Source: CAD feature listing. Evaluate the final solid. Frame: model axes, mm. A direction names the side the tool comes from. Give positions to 0.01 mm unless a question says otherwise; leave off trailing zeros. Order: outer loops, then holes, each group sorted by start corner. A loop starts at its lowest first (then second) coordinate and runs counter-clockwise, first axis right, second up. Notation, with made-up numbers: M -12,81.25 L 33,81.25 A18 cw 33,107.25 Z; hole C 45,89.5 d11. An arc over 180 degrees is marked long. Return JSON: item names as keys, results as strings.
from build123d import *

# Parameters (mm, degrees)
SKETCH1_R           = 4
BOSS_EXTRUDE1_DEPTH = 10
SKETCH2_W           = 2
SKETCH2_H           = 10
CUT_EXTRUDE1_DEPTH  = 10
SKETCH3_R           = 1.5
CUT_EXTRUDE2_DEPTH  = 10
SKETCH4_W           = 4
SKETCH4_H           = 9
CUT_EXTRUDE3_DEPTH  = 10
SKETCH5_W           = 30
SKETCH5_H           = 10
BOSS_EXTRUDE2_DEPTH = 5
SKETCH6_R           = 8
CUT_EXTRUDE4_DEPTH  = 48
SKETCH7_R           = 6
CUT_EXTRUDE5_DEPTH  = 65
SKETCH8_R           = 6
CUT_EXTRUDE6_DEPTH  = 16
BOSS_EXTRUDE3_DEPTH = 15
SKETCH10_R          = 6
CUT_EXTRUDE7_DEPTH  = 6
FILLET1_R           = 5
FILLET2_R           = 5


with BuildPart() as part:
    # Sketch1 → Boss-Extrude1 (new body)
    with BuildSketch(Plane.XY):
        Polygon((0, 0), (30, 0), (30, -84), (-35, -84), (-35, -52), (0, -52), align=None)
        with Locations((20, -39)):
            Circle(SKETCH1_R, mode=Mode.SUBTRACT)
        with Locations((20, -67)):
            Circle(SKETCH1_R, mode=Mode.SUBTRACT)
    extrude(amount=BOSS_EXTRUDE1_DEPTH)

    # Sketch2 → Cut-Extrude1 (cut)
    with BuildSketch(Plane.XY.offset(10)):
        with Locations((29, -15)):
            Rectangle(SKETCH2_W, SKETCH2_H)
    extrude(amount=-CUT_EXTRUDE1_DEPTH, mode=Mode.SUBTRACT)

    # Sketch3 → Cut-Extrude2 (cut)
    with BuildSketch(Plane(origin=(30, 0, 0), x_dir=(0, 0, -1), z_dir=(1, 0, 0))):
        with Locations(Location((-5, -5, 0), (0, 0, 90))):
            Circle(SKETCH3_R)
        with Locations(Location((-5, -25, 0), (0, 0, 90))):
            Circle(SKETCH3_R)
    extrude(amount=-CUT_EXTRUDE2_DEPTH, mode=Mode.SUBTRACT)

    # Sketch4 → Cut-Extrude3 (cut)
    with BuildSketch(Plane.XY.offset(10)):
        with Locations((22, -5)):
            Rectangle(SKETCH4_W, SKETCH4_H)
        with Locations((22, -25)):
            Rectangle(SKETCH4_W, SKETCH4_H)
    extrude(amount=-CUT_EXTRUDE3_DEPTH, mode=Mode.SUBTRACT)

    # Sketch5 → Boss-Extrude2 (add)
    with BuildSketch(Plane(origin=(0, 0, 0), x_dir=(1, 0, 0), z_dir=(0, 1, 0))):
        with Locations((15, -5)):
            Rectangle(SKETCH5_W, SKETCH5_H)
    extrude(amount=BOSS_EXTRUDE2_DEPTH)

    # Sketch6 → Cut-Extrude4 (cut)
    with BuildSketch(Plane.ZY.offset(35)):
        with Locations((0, -68)):
            Circle(SKETCH6_R)
    extrude(amount=-CUT_EXTRUDE4_DEPTH, mode=Mode.SUBTRACT)

    # Sketch7 → Cut-Extrude5 (cut)
    with BuildSketch(Plane(origin=(0, 5, 0), x_dir=(1, 0, 0), z_dir=(0, 1, 0))):
        with Locations((7, 0)):
            Circle(SKETCH7_R)
    extrude(amount=-CUT_EXTRUDE5_DEPTH, mode=Mode.SUBTRACT)

    # Sketch8 → Cut-Extrude6 (cut)
    with BuildSketch(Plane(origin=(0, -60, 0), x_dir=(1, 0, 0), z_dir=(0, 1, 0))):
        with Locations((7, 0)):
            Circle(SKETCH8_R)
    extrude(amount=-CUT_EXTRUDE6_DEPTH, mode=Mode.SUBTRACT)

    # Sketch9 → Boss-Extrude3 (add)
    with BuildSketch(Plane(origin=(0, 5, 0), x_dir=(1, 0, 0), z_dir=(0, 1, 0))):
        with BuildLine():
            Line((13, 0), (1, 0))
            ThreePointArc((1, 0), (7, -6), (13, 0))
        make_face()
    extrude(amount=-BOSS_EXTRUDE3_DEPTH)

    # Sketch10 → Cut-Extrude7 (cut)
    with BuildSketch(Plane(origin=(0, 0, 0), x_dir=(-1, 0, 0), z_dir=(0, 0, -1))):
        with Locations((-7, -10)):
            Circle(SKETCH10_R)
    extrude(amount=-CUT_EXTRUDE7_DEPTH, mode=Mode.SUBTRACT)

    # Fillet1
    fillet1_edges = [part.edges().sort_by_distance(p)[0] for p in [
        (-35, -52, 5),
    ]]
    fillet(fillet1_edges, radius=FILLET1_R)

    # Fillet2
    fillet2_edges = [part.edges().sort_by_distance(p)[0] for p in [
        (0, 5, 5),
    ]]
    fillet(fillet2_edges, radius=FILLET2_R)


solid = part.part
1. Section query B-B (z = 1.25). State how many separate pieces and enclosed holes the cut face has, then the cut area to 3 significant figures.
Evaluation:
{"separate pieces": "1", "enclosed holes": "4", "area": "2,180 mm^2"}
2. First-contact query: pin 1 (1.5 mm diameter, centred on y = -40, z = 7, fed in from -X). Flat tip, straight axial feed; report the tip coordinate or a pass-through.
Evaluation:
{"pin 1": "stops at x = 0"}
3. Section query D-D (y = -18.5). Return loops of the section in (x, z).
Evaluation:
{"outline": "M 0,0 L 1,0 A6 cw 13,0 L 28,0 L 28,10 L 0,10 Z"}
4. Set-up query: faces 1 (the face through (29, -20, 5)), 2 (the face through (22, -20.5, 5)), 3 (the face through (13, -68, 3)), 4 (the face through (27.04, -26.5, 5.07)). Return all of +Z, -Z, +X, -X, +Y, -Y with unobstructed straight access to the full face (end or side cutting, diameter ignored); none if empty.
Evaluation:
{"face 1": "+Z, -Z, +X", "face 2": "+Z, -Z", "face 3": "-Z, -X", "face 4": "+X"}
5. Draft query along X for faces 5 (the face through (30, -3, 5)), 6 (the face through (7, -36, 6)), 7 (the face through (27.04, -6.5, 5.07)). Return one class per face: pulls with the +X half, pulls with the -X half, needs draft (parallel to the pull), parting line crosses it, or undercut.
Evaluation:
{"face 5": "pulls with the +X half", "face 6": "undercut", "face 7": "needs draft"}
6. Section query C-C (x = -26). Return loops of the section in (y, z).
Evaluation:
{"outline": "M -84,0 L -76,0 A8 cw -60,0 L -52,0 L -52,10 L -84,10 Z"}
7. Ray query, probe 1 along Z at (x, y) = (26.15, -5); probe 2 along X at (y, z) = (-21.5, 6.5); probe 3 along Y at (x, z) = (-28.5, 6). Return the intervals inside material, ascending.
Evaluation:
{"probe 1": "z = 0 to 3.5, 6.5 to 10", "probe 2": "x = 0 to 20, 24 to 30", "probe 3": "y = -84 to -73.29, -62.71 to -52"}
8. Section query A-A (y = -2.5). Return loops of the section in (x, z), then the cut area to 3 significant figures.
Evaluation:
{"outline": "M 0,0 L 20,0 L 20,10 L 0,10 Z; M 24,0 L 30,0 L 30,10 L 24,10 Z", "area": "260 mm^2"}
